Model file for the job. Use its own axes, mm. Face numbers are marked on the shaded views. A direction names the side the tool comes from. Give positions to 0.01 mm unless a question says otherwise; leave off trailing zeros. Loops run counter-clockwise (first coordinate to the right, second up) from the corner with the lowest first, then second, coordinate; pieces in that order, holes last. Notation, with made-up numbers: M -20.5,-15 L 1.5,-15 A32 cw 1.5,20 Z; hole C 78.25,23.25 d7. An arc over 180 degrees is marked long. Answer in a Markdown table with one row per item.
```python
from build123d import *

# Parameters (mm, degrees)
F1_DEPTH = 25.4
F2_R     = 1.5875
F3_DEPTH = 25.4


with BuildPart() as f1:
    # F0 (on Top) → F1 (new body)
    with BuildSketch(Plane.XY):
        Polygon((-50.8, 0), (0, 0), (45.948514, 45.948514), (58.648514, 45.948514), (58.648514, 58.140514), (43.408514, 58.140514), (0, 14.732), (-50.8, 14.732), (-50.8, 9.652), (-25.4, 9.652), (-25.4, 5.08), (-50.8, 5.08), align=None)
    extrude(amount=F1_DEPTH)

    # F2 (on face) → F3 (cut)
    with BuildSketch(Plane(origin=(0, 58.140514, 0), x_dir=(-1, 0, 0), z_dir=(0, 1, 0))):
        with Locations((-51.028514, 12.7)):
            Circle(F2_R)
    extrude(amount=-F3_DEPTH, mode=Mode.SUBTRACT)


solid = f1.part
```
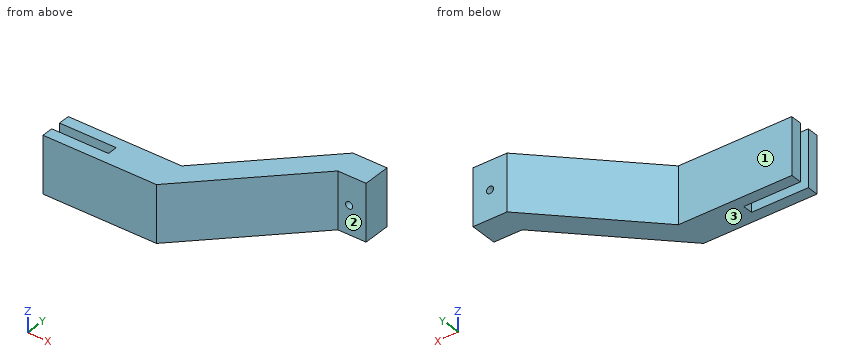
(1) Flat gauge pins, fed straight in: P1, Ø7.5, axis at x = -40.5, z = 18.5, coming from the +Y side; P2, Ø2.5, axis at y = 8, z = 8, coming from the -X side; P3, Ø10, axis at x = 52.5, z = 16, coming from the -Y side. Where does each tip first touch, or does it go through?
Established:
| item | result |
|---|---|
| P1 | stops at y = 14.73 |
| P2 | stops at x = -25.4 |
| P3 | stops at y = 45.95 |
(2) Saw through at A-A, the plane z = 12.7. Give the cut face in (x, y).
Established:
| item | result |
|---|---|
| outline | M -50.8,0 L 0,0 L 45.95,45.95 L 49.44,45.95 L 49.44,58.14 L 43.41,58.14 L 0,14.73 L -50.8,14.73 L -50.8,9.65 L -25.4,9.65 L -25.4,5.08 L -50.8,5.08 Z; M 52.62,45.95 L 58.65,45.95 L 58.65,58.14 L 52.62,58.14 Z |
(3) Saw through at B-B, the plane x = -39. Give the cut face in (y, z).
Established:
| item | result |
|---|---|
| outline | M 0,0 L 5.08,0 L 5.08,25.4 L 0,25.4 Z; M 9.65,0 L 14.73,0 L 14.73,25.4 L 9.65,25.4 Z |
(4) Saw through at D-D, the plane x = -17. Give the cut face in (y, z).
Established:
| item | result |
|---|---|
| outline | M 0,0 L 14.73,0 L 14.73,25.4 L 0,25.4 Z |
(5) Saw through at C-C, the plane z = 3.25. Give the cut face in (x, y), and give its area (3 significant figures).
Established:
| item | result |
|---|---|
| outline | M -50.8,0 L 0,0 L 45.95,45.95 L 58.65,45.95 L 58.65,58.14 L 43.41,58.14 L 0,14.73 L -50.8,14.73 L -50.8,9.65 L -25.4,9.65 L -25.4,5.08 L -50.8,5.08 Z |
| area | 1,460 mm2 |
(6) Wall check: L1, parallel to Y at x = 51, z = 23.5; L2, parallel to Y at x = -8, z = 12.25; L3, parallel to Y at x = -27, z = 23.75. Give the ranges that are in metal, low to high.
Established:
| item | result |
|---|---|
| L1 | y = 45.95 to 58.14 |
| L2 | y = 0 to 14.73 |
| L3 | y = 0 to 5.08, 9.65 to 14.73 |
(7) Which spindle directions (+Z, -Z, +X, -X, +Y, -Y) get a long thin tool onto all of the face, cutting with end or side? Do the marked faces 1, 2 and 3. Say none if no direction does.
Established:
| item | result |
|---|---|
| face 1 | +Z, -Z, -X, +Y |
| face 2 | +Z, -Z, +X, -Y |
| face 3 | -Z, +X, -X, +Y, -Y |
